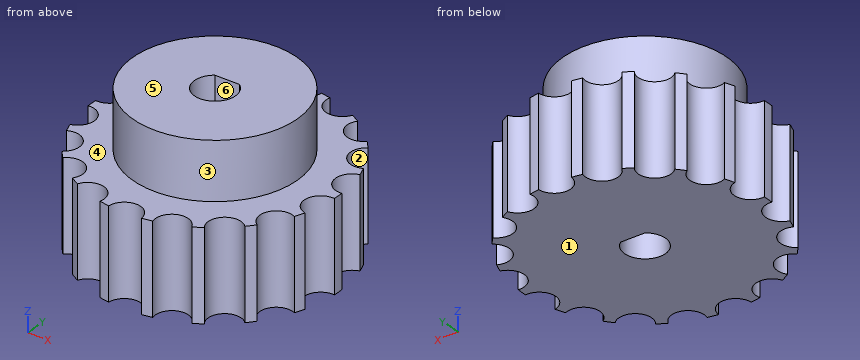
from build123d import *

# Parameters (mm, degrees)
SKETCH1_R           = 15
BOSS_EXTRUDE1_DEPTH = 11
SKETCH2_R           = 2
CUT_EXTRUDE1_DEPTH  = 11
SKETCH3_R           = 2.5
CUT_EXTRUDE2_DEPTH  = 11
BOSS_EXTRUDE2_START = 7
SKETCH5_R           = 10
SKETCH5_R_2         = 2.5
BOSS_EXTRUDE2_DEPTH = 7
BOSS_EXTRUDE3_DEPTH = 18


with BuildPart() as part:
    # Sketch1 → Boss-Extrude1 (new body)
    with BuildSketch(Plane.XY):
        Circle(SKETCH1_R)
    extrude(amount=BOSS_EXTRUDE1_DEPTH)

    # Sketch2 → Cut-Extrude1 (cut)
    with BuildSketch(Plane.XY.offset(11)):
        with Locations((0, 15)):
            Circle(SKETCH2_R)
        with Locations((5.13030215, 14.095389312)):
            Circle(SKETCH2_R)
        with Locations((9.641814145, 11.490666647)):
            Circle(SKETCH2_R)
        with Locations((12.990381057, 7.5)):
            Circle(SKETCH2_R)
        with Locations((14.772116295, 2.604722665)):
            Circle(SKETCH2_R)
        with Locations((14.772116295, -2.604722665)):
            Circle(SKETCH2_R)
        with Locations((12.990381057, -7.5)):
            Circle(SKETCH2_R)
        with Locations((9.641814145, -11.490666647)):
            Circle(SKETCH2_R)
        with Locations((5.13030215, -14.095389312)):
            Circle(SKETCH2_R)
        with Locations((0, -15)):
            Circle(SKETCH2_R)
        with Locations((-5.13030215, -14.095389312)):
            Circle(SKETCH2_R)
        with Locations((-9.641814145, -11.490666647)):
            Circle(SKETCH2_R)
        with Locations((-12.990381057, -7.5)):
            Circle(SKETCH2_R)
        with Locations((-14.772116295, -2.604722665)):
            Circle(SKETCH2_R)
        with Locations((-14.772116295, 2.604722665)):
            Circle(SKETCH2_R)
        with Locations((-12.990381057, 7.5)):
            Circle(SKETCH2_R)
        with Locations((-9.641814145, 11.490666647)):
            Circle(SKETCH2_R)
        with Locations((-5.13030215, 14.095389312)):
            Circle(SKETCH2_R)
    extrude(amount=-CUT_EXTRUDE1_DEPTH, mode=Mode.SUBTRACT)

    # Sketch3 → Cut-Extrude2 (cut)
    with BuildSketch(Plane.XY.offset(11)):
        Circle(SKETCH3_R)
    extrude(amount=-CUT_EXTRUDE2_DEPTH, mode=Mode.SUBTRACT)

    # Sketch5 → Boss-Extrude2 (add)
    with BuildSketch(Plane.XY.offset(11).offset(BOSS_EXTRUDE2_START)):
        Circle(SKETCH5_R)
        Circle(SKETCH5_R_2, mode=Mode.SUBTRACT)
    extrude(amount=-BOSS_EXTRUDE2_DEPTH)

    # Sketch6 → Boss-Extrude3 (add)
    with BuildSketch(Plane.XY.offset(18)):
        with BuildLine():
            Line((1.5, 2), (-1.5, 2))
            ThreePointArc((-1.5, 2), (0, 2.5), (1.5, 2))
        make_face()
    extrude(amount=-BOSS_EXTRUDE3_DEPTH)


solid = part.part
The listing builds one solid part. Answer for the finished solid, in the listing's coordinates (mm). Face numbers are marked on the shaded views. A direction names the side the tool comes from. Coordinates: 2 decimals unless noted, no trailing zeros. Write each loop counter-clockwise with the first axis right and the second up, starting at its lowest first coordinate (ties: lowest second). Pieces come first, ordered by that corner, then holes. Notation, with made-up numbers: (40.25, 1) - (70.25, 1) arc R19 ccw to (70.25, 28) - close; hole circle Ø2 at (-3.75, 48). An arc over 180 degrees is marked (long way). Return JSON: item names as keys, results as strings.
1. Which of the six approach directions +Z, -Z, +X, -X, +Y, -Y give full straight-line access (tool end or side, diameter ignored) to the marked faces 4, 5 and 6?
Final values:
{"face 4": "+Z", "face 5": "+Z, +X, -X, +Y, -Y", "face 6": "+Z, -Z"}
2. The part is cut by section C-C on z = 16.25. Determine the outline of the cut face in (x, y).
Final values:
{"outline": "circle Ø20 at (0, 0); hole (-1.5, 2) arc R2.5 ccw (long way) to (1.5, 2) - close"}
3. The part is cut by section D-D on y = -7.5. Determine the outline of the cut face in (x, z), then the cut area to 3 significant figures.
Final values:
{"outline": "(-10.99, 0) - (10.99, 0) - (10.99, 11) - (6.61, 11) - (6.61, 18) - (-6.61, 18) - (-6.61, 11) - (-10.99, 11) - close", "area": "334 mm^2"}
4. Each of these flat-tipped pins is pushed along its axis until it touches: pin 1 Ø2 at (x, y) = (8.5, -2) entering from -Z; pin 2 Ø3 at (x, y) = (0, 0) entering from -Z; pin 3 Ø1 at (x, z) = (-7, 5) entering from +Y; pin 4 Ø6 at (x, y) = (-10.5, 10.5) entering from +Z. Where does it stop, or does it pass through?
Final values:
{"pin 1": "z = 0", "pin 2": "through", "pin 3": "y = 13.29", "pin 4": "z = 11"}
5. The part is cut by section A-A on x = 0. Determine the outline of the cut face in (y, z).
Final values:
{"outline": "(-13, 0) - (-2.5, 0) - (-2.5, 18) - (-10, 18) - (-10, 11) - (-13, 11) - close; (2, 0) - (13, 0) - (13, 11) - (10, 11) - (10, 18) - (2, 18) - close"}
6. Consider line 1 along Y through (x, z) = (0, 4); line 2 along X through (y, z) = (-12.75, 9); line 3 along Y through (x, z) = (0, 14). Determine where each line is inside the solid, lowest interval first.
Final values:
{"line 1": "-13 to -2.5, 2 to 13", "line 2": "-7.9 to -6.61, -3.65 to 3.65, 6.61 to 7.9", "line 3": "-10 to -2.5, 2 to 10"}
7. The part is cut by section B-B on y = 0. Determine the outline of the cut face in (x, z).
Final values:
{"outline": "(-15, 0) - (-2.5, 0) - (-2.5, 18) - (-10, 18) - (-10, 11) - (-15, 11) - close; (2.5, 0) - (15, 0) - (15, 11) - (10, 11) - (10, 18) - (2.5, 18) - close"}
8. For a pull along X with two mould halves and no side action, classify the marked faces 1, 2 and 3 as +X half, -X half, draft (parallel to the pull), parting line (faces both ways), or undercut.
Final values:
{"face 1": "draft", "face 2": "undercut", "face 3": "parting line"}
